The listing builds one solid part. Answer for the finished solid, in the listing's coordinates (mm). Give positions to 0.01 mm unless a question says otherwise; leave off trailing zeros. Loops run counter-clockwise (first coordinate to the right, second up) from the corner with the lowest first, then second, coordinate; pieces in that order, holes last. Notation, with made-up numbers: (1.5, 14.25) -> (12.5, 14.25) arc R9 ccw to (12.5, 24.25) -> close; hole circle Ø3 at (30.5, 72). An arc over 180 degrees is marked (long way). One line per question, with ' | ' between items. Start each with the question number.
from build123d import *

# Parameters (mm, degrees)
SKETCH1_W           = 7.5
SKETCH1_H           = 26.881
SKETCH1_R           = 1.35
BOSS_EXTRUDE1_DEPTH = 2


with BuildPart() as part:
    # Sketch1 → Boss-Extrude1 (new body)
    with BuildSketch(Plane.XY):
        with Locations((0.25, -1.0005)):
            Rectangle(SKETCH1_W, SKETCH1_H)
        Circle(SKETCH1_R, mode=Mode.SUBTRACT)
    extrude(amount=BOSS_EXTRUDE1_DEPTH)


solid = part.part
1. The part is cut by section A-A (x = 0). Write down the section's boundary in (y, z), plus the area to 3 significant figures.
2. The part is cut by section C-C (z = 0.4). Write down the section's boundary in (x, y), plus the area to 3 significant figures.
3. Determine the mould class of faces 1 (the flat face through (-3.5, -1, 1)), 2 (the flat face through (2, -1, 0)), 3 (the cylindrical face through (-0.29, -1.32, 0.99)) for opening direction X: released by +X, released by -X, zero draft, split by the parting line, or undercut.
4. A straight line is drawn through the part: L1, parallel to Y at x = 0, z = 0.95. Find the intervals that lie inside material, in ascending order.
5. The part is cut by section B-B (y = 0). Write down the section's boundary in (x, z), plus the area to 3 significant figures.
Check sheet entries:
1) outline: (-14.44, 0) -> (-1.35, 0) -> (-1.35, 2) -> (-14.44, 2) -> close; (1.35, 0) -> (12.44, 0) -> (12.44, 2) -> (1.35, 2) -> close | area: 48.4 mm^2
2) outline: (-3.5, -14.44) -> (4, -14.44) -> (4, 12.44) -> (-3.5, 12.44) -> close; hole circle Ø2.7 at (0, 0) | area: 196 mm^2
3) face 1: released by -X | face 2: zero draft | face 3: undercut
4) L1: y = -14.44 to -1.35, 1.35 to 12.44
5) outline: (-3.5, 0) -> (-1.35, 0) -> (-1.35, 2) -> (-3.5, 2) -> close; (1.35, 0) -> (4, 0) -> (4, 2) -> (1.35, 2) -> close | area: 9.60 mm^2
